Work out the finished part from the listing and answer in its coordinate system (mm). A direction names the side the tool comes from. Coordinates: 2 decimals unless noted, no trailing zeros. Write each loop counter-clockwise with the first axis right and the second up, starting at its lowest first coordinate (ties: lowest second). Pieces come first, ordered by that corner, then holes. Notation, with made-up numbers: M 76.25,63 L 127.25,63 A10 ccw 127.25,74 Z; hole C -32.5,-31.5 d11. An arc over 180 degrees is marked long. Answer as CSV lines item,"result". Start each with the question number.
(1) A cutting plane is placed at B-B on x = 0. Give the vertices of the cut face in (y, z).
(2) Flat-ended cylindrical pins translate along their axes: P1, Ø4, axis at x = 29.5, y = -3.5, coming from the -Z side (3 decimals); P2, Ø8, axis at x = -16, y = 7, coming from the +Z side; P3, Ø15.5, axis at y = -12.5, z = -0.5, coming from the -X side. Find the tip coordinate at first contact, or state that the pin passes through.
(3) A cutting plane is placed at D-D on x = 18.5. Give the vertices of the cut face in (y, z).
(4) A cutting plane is placed at A-A on y = -6.5. Give the vertices of the cut face in (x, z) (3 decimals), then the cut area to 3 significant figures.
(5) Find the intervals of material crossed by L1, parallel to Y at x = 28, z = 0 (3 decimals); L2, parallel to Y at x = 16.5, z = -22; L3, parallel to Z at x = 28, y = -12 (3 decimals), in increasing order. Write a range as [from, to].
(6) A cutting plane is placed at C-C on y = 4.5. Give the vertices of the cut face in (x, z).
(7) For faces 1 (the cylindrical face through (-29.246, -19.683, -0.154)), 2 (the flat face through (8.245, 13.988, 7.325)), 3 (the flat face through (-26.67, -10, 0)), 4 (the flat face through (29, -6, 6.985)), 5 (the flat face through (29, -6, -6.985)), determine the directions among +Z, -Z, +X, -X, +Y, -Y from which every point of the face is accessible in a straight line to the end or side of a thin tool.
(8) The mould has two halves that part along X. Classify faces 6 (the cylindrical face through (15.456, 11.377, 20.157)), 7 (the flat face through (-31.75, -10, 0)), 8 (the flat face through (26.67, -10, 0)), 9 (the flat face through (-29, -6, 6.985)): released by +X, released by -X, zero draft, split by the parting line, or undercut.
from build123d import *

# Parameters (mm, degrees)
SKETCH1_R           = 50.8
BOSS_EXTRUDE1_DEPTH = 7.62
SKETCH2_W           = 5.08
SKETCH2_H           = 13.97
BOSS_EXTRUDE2_DEPTH = 12.7
SKETCH3_R           = 6.985
BOSS_EXTRUDE3_DEPTH = 5.08
SKETCH4_R           = 2.516115175
CUT_EXTRUDE1_DEPTH  = 5.08
SKETCH5_W           = 5.08
SKETCH5_H           = 13.97
BOSS_EXTRUDE4_DEPTH = 12.7
BOSS_EXTRUDE5_START = -5.08
SKETCH6_R           = 6.985
BOSS_EXTRUDE5_DEPTH = 5.08
SKETCH8_R           = 2.54
CUT_EXTRUDE2_DEPTH  = 5.08
SKETCH9_R           = 25.4
BOSS_EXTRUDE6_DEPTH = 7.62
CUT_EXTRUDE3_DEPTH  = 2.54


with BuildPart() as part:
    # Sketch1 → Boss-Extrude1 (new body)
    with BuildSketch(Plane(origin=(0, 0, 0), x_dir=(1, 0, 0), z_dir=(0, 1, 0))):
        with Locations(Location((0, 0, 0), (0, 0, 90))):
            Circle(SKETCH1_R)
    extrude(amount=BOSS_EXTRUDE1_DEPTH)

    # Sketch2 → Boss-Extrude2 (add)
    with BuildSketch(Plane.XZ):
        with Locations((-29.21, 0)):
            Rectangle(SKETCH2_W, SKETCH2_H)
    extrude(amount=BOSS_EXTRUDE2_DEPTH)

    # Sketch3 → Boss-Extrude3 (add)
    with BuildSketch(Plane.ZY.offset(31.75)):
        with Locations((0, -12.7)):
            Circle(SKETCH3_R)
    extrude(amount=-BOSS_EXTRUDE3_DEPTH)

    # Sketch4 → Cut-Extrude1 (cut)
    with BuildSketch(Plane.ZY.offset(31.75)):
        with Locations((0, -12.7)):
            Circle(SKETCH4_R)
    extrude(amount=-CUT_EXTRUDE1_DEPTH, mode=Mode.SUBTRACT)

    # Sketch5 → Boss-Extrude4 (add)
    with BuildSketch(Plane.XZ):
        with Locations((29.21, 0)):
            Rectangle(SKETCH5_W, SKETCH5_H)
    extrude(amount=BOSS_EXTRUDE4_DEPTH)

    # Sketch6 → Boss-Extrude5 (add)
    with BuildSketch(Plane(origin=(31.75, 0, 0), x_dir=(0, 0, -1), z_dir=(1, 0, 0)).offset(BOSS_EXTRUDE5_START)):
        with Locations((0, -12.7)):
            Circle(SKETCH6_R)
    extrude(amount=BOSS_EXTRUDE5_DEPTH)

    # Sketch8 → Cut-Extrude2 (cut)
    with BuildSketch(Plane(origin=(31.75, 0, 0), x_dir=(0, 0, -1), z_dir=(1, 0, 0))):
        with Locations((0, -12.7)):
            Circle(SKETCH8_R)
    extrude(amount=-CUT_EXTRUDE2_DEPTH, mode=Mode.SUBTRACT)

    # Sketch9 → Boss-Extrude6 (add)
    with BuildSketch(Plane(origin=(0, 7.62, 0), x_dir=(1, 0, 0), z_dir=(0, 1, 0))):
        with Locations(Location((0, 0, 0), (0, 0, 90))):
            Circle(SKETCH9_R)
    extrude(amount=BOSS_EXTRUDE6_DEPTH)

    # Sketch10 → Cut-Extrude3 (cut)
    with BuildSketch(Plane(origin=(0, 15.24, 0), x_dir=(1, 0, 0), z_dir=(0, 1, 0))):
        Polygon((1.37873117, -14.858671092), (-14.9225, 0), (-1.37873117, 14.858671092), (14.9225, 0), align=None)
    extrude(amount=-CUT_EXTRUDE3_DEPTH, mode=Mode.SUBTRACT)


solid = part.part
Here are the results:
1,outline,"M 0,-50.8 L 7.62,-50.8 L 7.62,-25.4 L 15.24,-25.4 L 15.24,-13.6 L 12.7,-13.6 L 12.7,13.6 L 15.24,13.6 L 15.24,25.4 L 7.62,25.4 L 7.62,50.8 L 0,50.8 Z"
2,P1,"stops at z = -6.985"
2,P2,"stops at z = 49.36"
2,P3,"stops at x = -31.75"
3,outline,"M 0,-47.31 L 7.62,-47.31 L 7.62,-17.4 L 15.24,-17.4 L 15.24,17.4 L 7.62,17.4 L 7.62,47.31 L 0,47.31 Z"
4,outline,"M -31.75,-6.985 L -26.67,-6.985 L -26.67,6.985 L -31.75,6.985 Z; M 26.67,-6.985 L 31.75,-6.985 L 31.75,6.985 L 26.67,6.985 Z"
4,area,"142 mm^2"
5,L1,"y = [-19.685, -15.24], [-10.16, 7.62]"
5,L2,"y = [0, 7.62]"
5,L3,"z = [-6.985, -2.442], [2.442, 6.985]"
6,outline,"C 0,0 d101.6"
7,face 1,"+X, -X, -Y"
7,face 2,"+Y"
7,face 3,"+Z, -Z, -Y"
7,face 4,"+Z, +X, -X, -Y"
7,face 5,"-Z, +X, -X, -Y"
8,face 6,"split by the parting line"
8,face 7,"released by -X"
8,face 8,"undercut"
8,face 9,"zero draft"
